```python
from build123d import *


with BuildPart() as f1:
    # F0 (on Front) → F1 (revolve)
    with BuildSketch(Plane.XZ):
        with BuildLine():
            Line((21, 0), (24, 0))
            Line((24, 0), (24, 1.865))
            Line((24, 1.865), (25.088, 1.865))
            ThreePointArc((25.088, 1.865), (22.102986, 4.890684), (18, 6))
            Line((18, 6), (0, 6))
            Line((0, 6), (0, 4))
            Line((0, 4), (22, 4))
            Line((22, 4), (22, 1))
            Line((22, 1), (21, 1))
            Line((21, 1), (21, 0))
        make_face()
        with BuildLine():
            Line((24, 1.865), (24, 0))
            ThreePointArc((24, 0), (25.07958, 0.620055), (25.088, 1.865))
            Line((25.088, 1.865), (24, 1.865))
        make_face()
    revolve(axis=Axis((0, 0, 5), (0, 0, 1)))


solid = f1.part
```
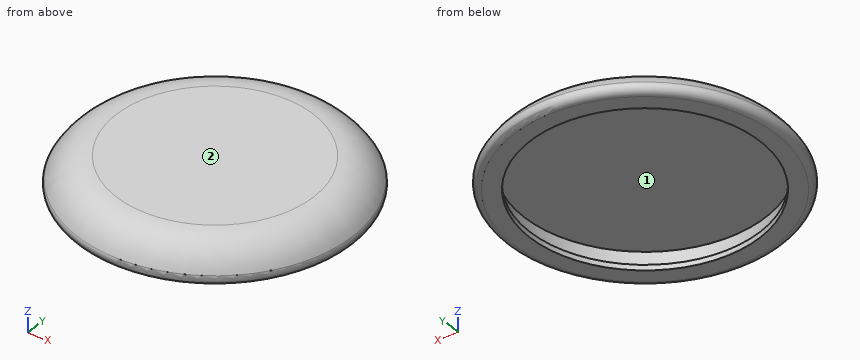
Can you work these out from the model? Positions are in its coordinate system, mm. Face numbers are marked on the shaded views. Round coordinates to 2 decimals unless told otherwise and drop trailing zeros. Loops run counter-clockwise (first coordinate to the right, second up) from the corner with the lowest first, then second, coordinate; pieces in that order, holes last.
Item 1: Suppose I cut it at C-C, the plane z = 5.25. Write out the boundary of the cut face in (x, y).
Item 2: Please list where these lines run through material, in increasing order: L1, parallel to Z at x = -1, y = -15.5; L2, parallel to X at y = 10.5, z = 2; L3, parallel to Y at x = -10, z = 2.5.
Item 3: Will these pins go through, and if not, where does the flat tip stop? pin 1 Ø2 at (x, z) = (14.5, 1) entering from -Y; pin 2 Ø13 at (x, y) = (-5, 5.5) entering from -Z; pin 3 Ø2 at (x, z) = (-9.5, 5) entering from +Y.
Item 4: If we mould it in two halves opening along X, with no side actions, what happens to the marked faces 1 and 2? For each: +X half, -X half, draft (parallel to the pull), parting line (faces both ways), or undercut.
Item 5: Suppose I cut it at A-A, the plane y = 0. Write out the boundary of the cut face in (x, z) (3 decimals).
Reported:
1. outline: circle Ø42.83 at (0, 0)
2. L1: z = 4 to 6
2. L2: x = -22.7 to -19.33, 19.33 to 22.7
2. L3: y = -22.57 to -19.6, 19.6 to 22.57
3. pin 1: stops at y = -21.33
3. pin 2: stops at z = 4
3. pin 3: stops at y = 21.4
4. face 1: undercut
4. face 2: draft
5. outline: (-25.088, 1.865) arc R1.25 ccw to (-24, 0) - (-21, 0) - (-21, 1) - (-22, 1) - (-22, 4) - (22, 4) - (22, 1) - (21, 1) - (21, 0) - (24, 0) arc R1.25 ccw to (25.088, 1.865) arc R8.142 ccw to (18, 6) - (-18, 6) arc R8.142 ccw to start
